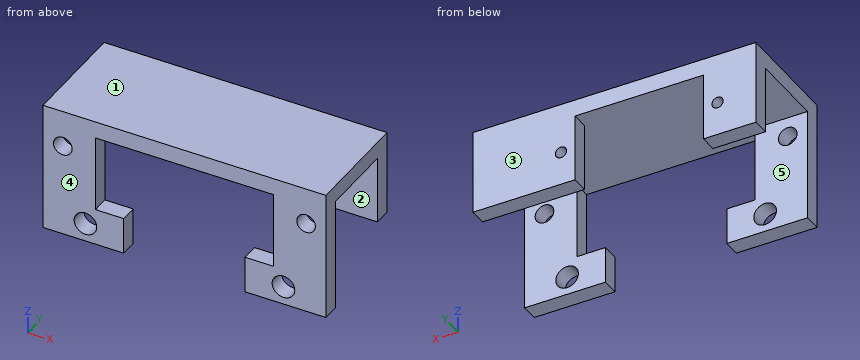
```python
from build123d import *

# Parameters (mm, degrees)
SKETCH_1_W          = 50
SKETCH_1_H          = 19.4
EXTRUDE_1_DEPTH     = 3
SKETCH_2_W          = 18.05
SKETCH_2_H          = 3
SKETCH_2_W_2        = 9.27
EXTRUDE_3_DEPTH     = 12
SKETCH_5_R          = 1
CUT_EXTRUDE_1_DEPTH = 4
SKETCH_6_W          = 9.27
SKETCH_6_H          = 2.996679997
EXTRUDE_5_DEPTH     = 20
SKETCH_9_W          = 6.5
SKETCH_9_H          = 2.996679997
EXTRUDE_6_DEPTH     = 5
SKETCH_10_W         = 6.5
SKETCH_10_H         = 2.996679997
EXTRUDE_7_DEPTH     = 5
SKETCH_11_R         = 2
SKETCH_11_R_2       = 1.65
CUT_EXTRUDE_3_DEPTH = 5
SKETCH_12_R         = 2
SKETCH_12_R_2       = 1.65
CUT_EXTRUDE_4_DEPTH = 5


with BuildPart() as part:
    # 草图1 → 凸台-拉伸1 (new body)
    with BuildSketch(Plane.XY):
        with Locations((25, 9.7)):
            Rectangle(SKETCH_1_W, SKETCH_1_H)
    extrude(amount=EXTRUDE_1_DEPTH)

    # 草图2 → 凸台-拉伸3 (add)
    with BuildSketch(Plane(origin=(0, 0, 0), x_dir=(-1, 0, 0), z_dir=(0, 0, -1))):
        with Locations((-40.975, 17.9)):
            Rectangle(SKETCH_2_W, SKETCH_2_H)
        with Locations((-4.635, 17.9)):
            Rectangle(SKETCH_2_W_2, SKETCH_2_H)
    extrude(amount=EXTRUDE_3_DEPTH)

    # 草图5 → 切除-拉伸1 (cut)
    with BuildSketch(Plane(origin=(0, 19.4, 0), x_dir=(1, 0, 0), z_dir=(0, 1, 0))):
        with Locations((34.45, 6)):
            Circle(SKETCH_5_R)
        with Locations((6.78, 6)):
            Circle(SKETCH_5_R)
    extrude(amount=-CUT_EXTRUDE_1_DEPTH, mode=Mode.SUBTRACT)

    # 草图6 → 凸台-拉伸5 (add)
    with BuildSketch(Plane(origin=(0, 0, 0), x_dir=(-1, 0, 0), z_dir=(0, 0, -1))):
        with Locations((-45.365, 1.498339999)):
            Rectangle(SKETCH_6_W, SKETCH_6_H)
        with Locations((-4.635, 1.498339999)):
            Rectangle(SKETCH_6_W, SKETCH_6_H)
    extrude(amount=EXTRUDE_5_DEPTH)

    # 草图9 → 凸台-拉伸6 (add)
    with BuildSketch(Plane(origin=(9.27, 0, 0), x_dir=(0, 0, -1), z_dir=(1, 0, 0))):
        with Locations((16.75, 1.498339999)):
            Rectangle(SKETCH_9_W, SKETCH_9_H)
    extrude(amount=EXTRUDE_6_DEPTH)

    # 草图10 → 凸台-拉伸7 (add)
    with BuildSketch(Plane.ZY.offset(-40.73)):
        with Locations((-16.75, 1.498339999)):
            Rectangle(SKETCH_10_W, SKETCH_10_H)
    extrude(amount=EXTRUDE_7_DEPTH)

    # 草图11 → 切除-拉伸3 (cut)
    with BuildSketch(Plane(origin=(0, 2.996679997, 0), x_dir=(1, 0, 0), z_dir=(0, 1, 0))):
        with Locations((42.5, 16.75)):
            Circle(SKETCH_11_R)
        with Locations((46.5, 3.5)):
            Circle(SKETCH_11_R_2)
    extrude(amount=-CUT_EXTRUDE_3_DEPTH, mode=Mode.SUBTRACT)

    # 草图12 → 切除-拉伸4 (cut)
    with BuildSketch(Plane(origin=(0, 2.996679997, 0), x_dir=(1, 0, 0), z_dir=(0, 1, 0))):
        with Locations((7.5, 16.75)):
            Circle(SKETCH_12_R)
        with Locations((3.5, 3.5)):
            Circle(SKETCH_12_R_2)
    extrude(amount=-CUT_EXTRUDE_4_DEPTH, mode=Mode.SUBTRACT)


solid = part.part
```
Source: CAD feature listing. Evaluate the final solid. Frame: model axes, mm. Face numbers are marked on the shaded views. A direction names the side the tool comes from. Give positions to 0.01 mm unless a question says otherwise; leave off trailing zeros. Loops run counter-clockwise (first coordinate to the right, second up) from the corner with the lowest first, then second, coordinate; pieces in that order, holes last. Notation, with made-up numbers: (-18.75, 45.25) -> (27.25, 45.25) arc R23 cw to (27.25, 71.25) -> close; hole circle Ø2 at (-12.75, -36). An arc over 180 degrees is marked (long way). Put each result on its own line as item: value. Start each with the question number.
1) Cut plane C-C (z = -3.5). Return loops of the section in (x, y), then the cut area to 3 significant figures.
2) Material intervals for probe 1 along X at (y, z) = (1.5, -16.75); probe 2 along X at (y, z) = (2, -3.5); probe 3 along Z at (x, y) = (42.5, 1.3), sorted ascending.
3) Cut plane A-A (x = 34.45). Return loops of the section in (y, z), then the cut area to 3 significant figures.
4) Cut plane B-B (z = -16.75). Return loops of the section in (x, y).
5) Cut plane D-D (x = 6.78). Return loops of the section in (y, z).
6) Contact query for flat-ended pins moving along their axis: P1, Ø1.5, axis at x = 7, y = 17.5, coming from the -Z side; P2, Ø1, axis at x = 43.5, y = 14, coming from the -Z side. Output: stop coordinate, or through.
7) Draft query along Y for the marked faces 1, 2 and 3. Return one class per face: released by +Y, released by -Y, zero draft, split by the parting line, or undercut.
8) Reachability of the marked faces 4 and 5 from +Z, -Z, +X, -X, +Y, -Y: full face, straight path, thin tool, end or side. Return the list, or none.
Results are:
1. outline: (0, 0) -> (1.85, 0) -> (1.85, 3) -> (0, 3) -> close; (0, 16.4) -> (9.27, 16.4) -> (9.27, 19.4) -> (0, 19.4) -> close; (5.15, 0) -> (9.27, 0) -> (9.27, 3) -> (5.15, 3) -> close; (31.95, 16.4) -> (50, 16.4) -> (50, 19.4) -> (31.95, 19.4) -> close; (40.73, 0) -> (44.85, 0) -> (44.85, 3) -> (40.73, 3) -> close; (48.15, 0) -> (50, 0) -> (50, 3) -> (48.15, 3) -> close
1. area: 118 mm2
2. probe 1: x = 0 to 5.5, 9.5 to 14.27, 35.73 to 40.5, 44.5 to 50
2. probe 2: x = 0 to 1.85, 5.15 to 9.27, 40.73 to 44.85, 48.15 to 50
2. probe 3: z = -20 to -18.75, -14.75 to 3
3. outline: (0, 0) -> (16.4, 0) -> (16.4, -5) -> (19.4, -5) -> (19.4, 3) -> (0, 3) -> close; (16.4, -12) -> (19.4, -12) -> (19.4, -7) -> (16.4, -7) -> close
3. area: 88.2 mm2
4. outline: (0, 0) -> (5.5, 0) -> (5.5, 3) -> (0, 3) -> close; (9.5, 0) -> (14.27, 0) -> (14.27, 3) -> (9.5, 3) -> close; (35.73, 0) -> (40.5, 0) -> (40.5, 3) -> (35.73, 3) -> close; (44.5, 0) -> (50, 0) -> (50, 3) -> (44.5, 3) -> close
5. outline: (0, -20) -> (3, -20) -> (3, -18.62) -> (0, -18.62) -> close; (0, -14.88) -> (3, -14.88) -> (3, 0) -> (16.4, 0) -> (16.4, -5) -> (19.4, -5) -> (19.4, 3) -> (0, 3) -> close; (16.4, -12) -> (19.4, -12) -> (19.4, -7) -> (16.4, -7) -> close
6. P1: stops at z = -12
6. P2: stops at z = 0
7. face 1: zero draft
7. face 2: undercut
7. face 3: released by +Y
8. face 4: +Z, -Z, +X, -X, -Y
8. face 5: -Z, +X, -X
